```python
from build123d import *

# Parameters (mm, degrees)
SKETCH_1_W           = 7.62
SKETCH_1_H           = 6.35
EXTRUDE_1_DEPTH      = 5.08
SKETCH_2_W           = 6.62
SKETCH_2_H           = 5.35
CUT_EXTRUDE_1_DEPTH  = 4.08
SKETCH_3_W           = 2
SKETCH_3_H           = 4.08
CUT_EXTRUDE_2_DEPTH  = 1
EXTRUDE_2_DEPTH      = 2
EXTRUDE_2_DEPTH_BACK = 3.58
SKETCH_4_W           = 0.75
SKETCH_4_H           = 0.75


with BuildPart() as part:
    # 草图1 → 拉伸1 (new body)
    with BuildSketch(Plane(origin=(0, 0, 0), x_dir=(1, 0, 0), z_dir=(0, 1, 0))):
        Rectangle(SKETCH_1_W, SKETCH_1_H)
    extrude(amount=EXTRUDE_1_DEPTH)

    # 草图2 → 切除-拉伸1 (cut)
    with BuildSketch(Plane(origin=(0, 5.08, 0), x_dir=(-1, 0, 0), z_dir=(0, 1, 0))):
        Rectangle(SKETCH_2_W, SKETCH_2_H)
    extrude(amount=-CUT_EXTRUDE_1_DEPTH, mode=Mode.SUBTRACT)

    # 草图3 → 切除-拉伸2 (cut)
    with BuildSketch(Plane.XY.offset(3.175)):
        with Locations((0, 3.04)):
            Rectangle(SKETCH_3_W, SKETCH_3_H)
    extrude(amount=-CUT_EXTRUDE_2_DEPTH, mode=Mode.SUBTRACT)

    # 草图4 → 拉伸2 (add, two sides: drawn at the far end of the back side and taken through both)
    with BuildSketch(Plane.XZ.offset(-EXTRUDE_2_DEPTH_BACK)):
        with Locations((-1.27, 0.635)):
            Rectangle(SKETCH_4_W, SKETCH_4_H)
        with Locations((1.27, 0.635)):
            Rectangle(SKETCH_4_W, SKETCH_4_H)
    extrude(amount=EXTRUDE_2_DEPTH + EXTRUDE_2_DEPTH_BACK)


solid = part.part
```
Part model, mm, in its own coordinate system. A direction names the side the tool comes from. Round coordinates to 2 decimals unless told otherwise and drop trailing zeros. Write each loop counter-clockwise with the first axis right and the second up, starting at its lowest first coordinate (ties: lowest second). Pieces come first, ordered by that corner, then holes. Notation, with made-up numbers: M -40,32 L -7,32 A24 cw -7,70 Z; hole C -8,14.5 d7. An arc over 180 degrees is marked long. One line per question, with ' | ' between items.
(1) Pin check, flat tips, straight feed: pin 1 (0.6 mm diameter, centred on x = -1.5, z = 0.5, fed in from +Y); pin 2 (0.6 mm diameter, centred on x = -1, y = -1, fed in from -Z). Stop position of each tip, or through.
Answer key:
pin 1: stops at y = 3.58 | pin 2: stops at z = 0.26
(2) Saw through at A-A on y = -0.25. Write the cut outline in (x, z) (3 decimals).
Answer key:
outline: M -1.645,0.26 L -0.895,0.26 L -0.895,1.01 L -1.645,1.01 Z; M 0.895,0.26 L 1.645,0.26 L 1.645,1.01 L 0.895,1.01 Z
(3) Saw through at C-C on y = 2.5. Write the cut outline in (x, z) (3 decimals), then the cut area to 3 significant figures.
Answer key:
outline: M -3.81,-3.175 L 3.81,-3.175 L 3.81,3.175 L 1,3.175 L 1,2.675 L 3.31,2.675 L 3.31,-2.675 L -3.31,-2.675 L -3.31,2.675 L -1,2.675 L -1,3.175 L -3.81,3.175 Z; M -1.645,0.26 L -0.895,0.26 L -0.895,1.01 L -1.645,1.01 Z; M 0.895,0.26 L 1.645,0.26 L 1.645,1.01 L 0.895,1.01 Z | area: 13.1 mm^2
(4) Saw through at B-B on z = 3. Write the cut outline in (x, y), then the cut area to 3 significant figures.
Answer key:
outline: M -3.81,0 L 3.81,0 L 3.81,5.08 L 1,5.08 L 1,1 L -1,1 L -1,5.08 L -3.81,5.08 Z | area: 30.5 mm^2
(5) Two-plate mould, pull along X, no slides. Class faces 1 (the face through (3.31, 3, 0)), 2 (the face through (3.81, 3, 0)), 3 (the face through (-0.1, 0.8, 3.175)), 4 (the face through (0, 1, 0)): released by +X, released by -X, zero draft, split by the parting line, or undercut.
Answer key:
face 1: undercut | face 2: released by +X | face 3: zero draft | face 4: undercut
(6) Saw through at D-D on x = 2.75. Write the cut outline in (y, z) (3 decimals), then the cut area to 3 significant figures.
Answer key:
outline: M 0,-3.175 L 5.08,-3.175 L 5.08,-2.675 L 1,-2.675 L 1,2.675 L 5.08,2.675 L 5.08,3.175 L 0,3.175 Z | area: 10.4 mm^2
(7) Probe line 1 along Z through (x, y) = (-1.25, 2.5) (3 decimals); line 2 along X through (y, z) = (2, -1.25); line 3 along Z through (x, y) = (-3.25, 2.25) (3 decimals). List the from-to ranges inside material, lowest first.
Answer key:
line 1: z = -3.175 to -2.675, 0.26 to 1.01, 2.675 to 3.175 | line 2: x = -3.81 to -3.31, 3.31 to 3.81 | line 3: z = -3.175 to -2.675, 2.675 to 3.175
(8) 3-axis set-ups, long thin cutter, end or side, ignore diameter. For faces 5 (the face through (-3.81, 3, 0)), 6 (the face through (-3.31, 3, 0)): which of +Z, -Z, +X, -X, +Y, -Y reach the whole face in a straight line?
Answer key:
face 5: +Z, -Z, -X, +Y, -Y | face 6: +Y
